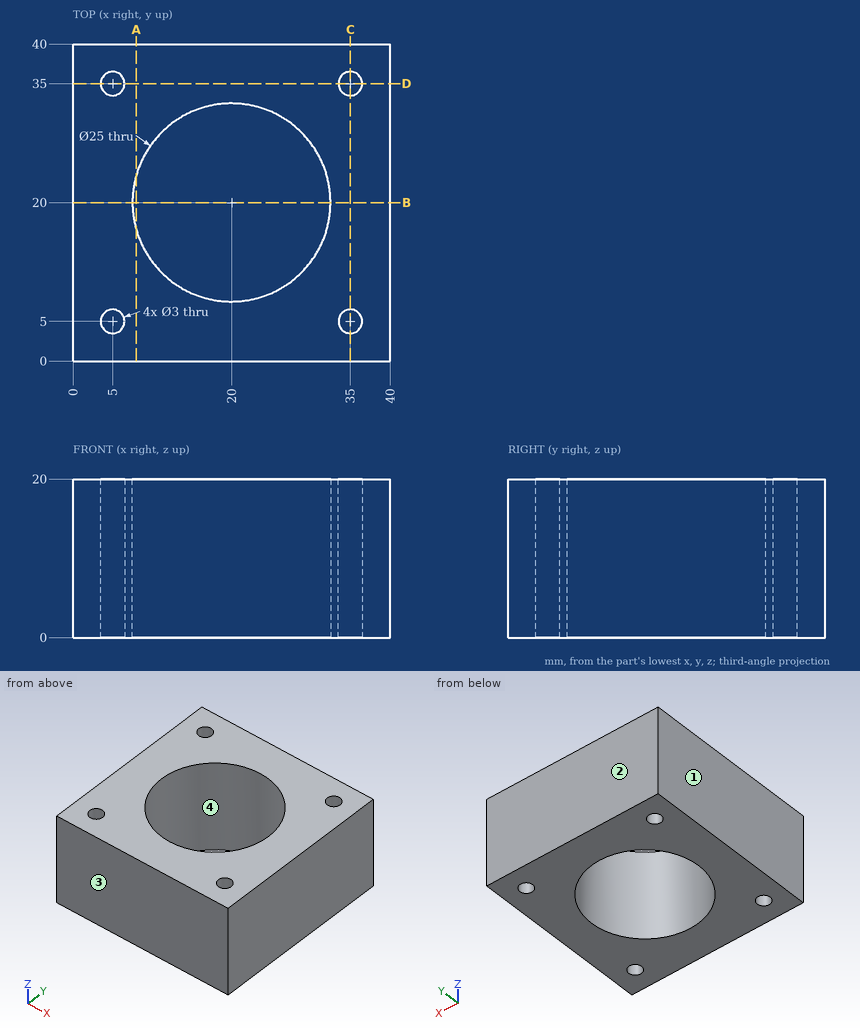
Answer from the drawing. Dimensions are ordinates in mm from the lowest x, y and z of the part. Give positions to 0.01 mm unless a question says otherwise; leave off trailing zeros. Order: outer loops, then holes, each group sorted by start corner. A loop starts at its lowest first (then second) coordinate and runs counter-clockwise, first axis right, second up. Notation, with made-up numbers: (-8, -18) -> (26, -18) arc R25 ccw to (26, 20) -> close; hole circle Ø8 at (-20, -2). An arc over 180 degrees is marked (long way). One line per item, written item: value. Start each with the question number.
(1) The part is cut by section C-C (x = 35). Determine the outline of the cut face in (y, z), and give its area (3 significant figures).
(2) Flat-ended cylindrical pins translate along their axes: P1, Ø3.5, axis at x = 5, y = 35, coming from the -Z side; P2, Ø10, axis at x = 18.5, y = 22.5, coming from the -Z side. Find the tip coordinate at first contact, or state that the pin passes through.
(3) The part is cut by section B-B (y = 20). Determine the outline of the cut face in (x, z).
(4) For a pull along Y with two mould halves and no side action, classify the marked faces 1, 2, 3 and 4 as released by +Y, released by -Y, zero draft, split by the parting line, or undercut.
(5) Straight lines are drawn through the part: L1, parallel to Y at x = 5, z = 15.5; L2, parallel to Y at x = 34, z = 9.75; L3, parallel to Y at x = 20, z = 16.25. For each, find the intervals that lie inside material, in ascending order.
(6) The part is cut by section A-A (x = 8). Determine the outline of the cut face in (y, z).
Taken from the geometry:
1. outline: (0, 0) -> (3.5, 0) -> (3.5, 20) -> (0, 20) -> close; (6.5, 0) -> (33.5, 0) -> (33.5, 20) -> (6.5, 20) -> close; (36.5, 0) -> (40, 0) -> (40, 20) -> (36.5, 20) -> close
1. area: 680 mm^2
2. P1: z = 0
2. P2: through
3. outline: (0, 0) -> (7.5, 0) -> (7.5, 20) -> (0, 20) -> close; (32.5, 0) -> (40, 0) -> (40, 20) -> (32.5, 20) -> close
4. face 1: zero draft
4. face 2: released by +Y
4. face 3: released by -Y
4. face 4: undercut
5. L1: 0 to 3.5, 6.5 to 33.5, 36.5 to 40
5. L2: 0 to 3.88, 6.12 to 33.88, 36.12 to 40
5. L3: 0 to 7.5, 32.5 to 40
6. outline: (0, 0) -> (16.5, 0) -> (16.5, 20) -> (0, 20) -> close; (23.5, 0) -> (40, 0) -> (40, 20) -> (23.5, 20) -> close
